Geometry check sheet. Reference: the model listing, model coordinates, mm. A direction names the side the tool comes from. Give positions to 0.01 mm unless a question says otherwise; leave off trailing zeros. Order: outer loops, then holes, each group sorted by start corner. A loop starts at its lowest first (then second) coordinate and runs counter-clockwise, first axis right, second up.
from build123d import *

# Parameters (mm, degrees)
F0_W     = 76.2
F0_H     = 76.2
F1_DEPTH = 3.175
F2_R     = 5.08
F4_DEPTH = 76.201
F5_R     = 2.54
F6_DEPTH = 25.4


with BuildPart() as f1:
    # F0 (on Top) → F1 (new body, symmetric)
    with BuildSketch(Plane.XY):
        Rectangle(F0_W, F0_H)
    extrude(amount=F1_DEPTH, both=True)

    # F2
    f2_edges = [f1.edges().sort_by_distance(p)[0] for p in [
        (38.1, -38.1, 0),
        (38.1, 38.1, 0),
        (-38.1, 38.1, 0),
        (-38.1, -38.1, 0),
    ]]
    fillet(f2_edges, radius=F2_R)

    # F3 (on face) → F4 (cut, through all)
    with BuildSketch(Plane.XZ.offset(38.1)):
        with BuildLine():
            Line((4.875244, 3.175), (-4.869716, 3.175))
            ThreePointArc((-4.869716, 3.175), (0.002764, -1e-06), (4.875244, 3.175))
        make_face()
    extrude(amount=-F4_DEPTH, mode=Mode.SUBTRACT)

    # F5 (on face) → F6 (join)
    with BuildSketch(Plane(origin=(0, 0, -3.175), x_dir=(1, 0, 0), z_dir=(0, 0, -1))):
        with Locations((33.02, -33.02)):
            Circle(F5_R)
    extrude(amount=F6_DEPTH)


solid = f1.part
Item 1: Set-up check for faces 1 (the flat face through (-38.1, 0, 0)), 2 (the cylindrical face through (31.15, 31.3, -15.7)): record each of +Z, -Z, +X, -X, +Y, -Y from which the full face is reachable in a straight line by a thin tool's end or side.
Reported:
face 1: +Z, -Z, -X, +Y, -Y
face 2: -Z
Item 2: Sectioned sample at B-B (x = 24). Enter the section's corners in (y, z) (3 decimals), and give its area (3 significant figures).
Reported:
outline: (-38.1, -3.175) - (38.1, -3.175) - (38.1, 3.175) - (-38.1, 3.175) - close
area: 484 mm2
Item 3: Sectioned sample at C-C (z = -9.5). Enter the section's corners in (x, y).
Reported:
outline: circle Ø5.08 at (33.02, 33.02)
Item 4: Sectioned sample at A-A (y = -22.5). Enter the section's corners in (x, z) (1 decimal).
Reported:
outline: (-38.1, -3.2) - (38.1, -3.2) - (38.1, 3.2) - (4.9, 3.2) arc R5.3 cw to (-4.9, 3.2) - (-38.1, 3.2) - close
Item 5: Scan lines: L1, parallel to Z at x = -12, y = -32.5 (3 decimals); L2, parallel to Y at x = 33, z = -21; L3, parallel to X at y = -6, z = 2. Record each from-to range of solid material in increasing order.
Reported:
L1: z = -3.175 to 3.175
L2: y = 30.48 to 35.56
L3: x = -38.1 to -4.16, 4.16 to 38.1
Item 6: Gauge pin test, flat ends, axial feed: pin 1 (4 mm diameter, centred on x = 2, y = 28, fed in from +Z); pin 2 (12 mm diameter, centred on x = -10.5, y = 4.5, fed in from -Z) (3 decimals). Record the tip position at first contact, or that the pin passes through.
Reported:
pin 1: stops at z = 1.81
pin 2: stops at z = -3.175
